```python
from build123d import *

# Parameters (mm, degrees)
BOSS_EXTRUDE1_DEPTH = 25.654
FILLET1_R           = 25.4
FILLET2_R           = 2.54


with BuildPart() as part:
    # Sketch1 → Boss-Extrude1 (new body)
    with BuildSketch(Plane(origin=(0, 0, 0), x_dir=(0, 0, -1), z_dir=(1, 0, 0))):
        Polygon((-8.1595, -12.7), (-6.1595, -12.7), (-6.1595, 0), (6.1595, 0), (6.1595, -25.4), (8.1595, -25.4), (8.1595, 3.175), (-8.1595, 3.175), align=None)
    extrude(amount=BOSS_EXTRUDE1_DEPTH)

    # Fillet1
    # the kernel refuses this fillet: 25.4 mm, written as the material it takes off along each edge
    with BuildSketch(Plane(origin=(-24.69817807, -12.7, 8.1595), x_dir=(0, 0, -1), z_dir=(1, 0, 0))) as fillet1_piece_1:
        with BuildLine():
            CenterArc((25.4, 9.879271228), FILLET1_R, 180, 22.889037196)
            Line((0, 9.879271228), (-0.508, 9.879271228))
            Line((-0.508, 9.879271228), (-0.508, 0))
            Line((-0.508, 0), (0, -0.508))
            ThreePointArc((0, -0.508), (1, -0.508), (1.532, -0.197585425))
            Line((1.532, -0.197585425), (2, 0))
        make_face()
    extrude(amount=75.050356141, mode=Mode.SUBTRACT)
    with BuildSketch(Plane(origin=(-24.69817807, -25.4, -8.1595), x_dir=(0, 0, 1), z_dir=(1, 0, 0))) as fillet1_piece_2:
        with BuildLine():
            CenterArc((25.4, -9.879271228), FILLET1_R, 157.110962804, 22.889037196)
            Line((0, -9.879271228), (-0.508, -9.879271228))
            Line((-0.508, -9.879271228), (-0.508, 0))
            Line((-0.508, 0), (0, 0.508))
            ThreePointArc((0, 0.508), (1, 0.508), (1.532, 0.197585425))
            Line((1.532, 0.197585425), (2, 0))
        make_face()
    extrude(amount=75.050356141, mode=Mode.SUBTRACT)

    # Fillet2
    fillet2_edges = [part.edges().sort_by_distance(p)[0] for p in [
        (12.827, 3.175, 8.1595),
        (12.827, 3.175, -8.1595),
    ]]
    fillet(fillet2_edges, radius=FILLET2_R)


solid = part.part
```
Geometry check sheet. Reference: the model listing, model coordinates, mm. A direction names the side the tool comes from. Round coordinates to 2 decimals unless told otherwise and drop trailing zeros. Order: outer loops, then holes, each group sorted by start corner. A loop starts at its lowest first (then second) coordinate and runs counter-clockwise, first axis right, second up. Notation, with made-up numbers: (77, -7.5) - (82, -7.5) arc R28 ccw to (82, 11.5) - close; hole circle Ø1 at (-32.75, -26.5). An arc over 180 degrees is marked (long way). Use a Markdown table: item, result. Add a question column.
1) Set-up check for faces 5 (the flat face through (13, -6, 6.16)), 6 (the cylindrical face through (13.007, 2.411, 7.435)): record each of +Z, -Z, +X, -X, +Y, -Y from which the full face is reachable in a straight line by a thin tool's end or side.
2) Section check C-C (y = -6.5). Record the cut outline in (x, z).
3) Thickness scan on line 1 along Z through (x, y) = (12.5, -3); line 2 along Z through (x, y) = (23.5, -8); line 3 along Y through (x, z) = (12.75, 5) (3 decimals). Record the ranges inside material, lowest first.
4) Section check D-D (z = 2.75). Record the cut outline in (x, y) (3 decimals).
5) Section check B-B (x = 8). Record the cut outline in (y, z) (1 decimal), then the cut area to 3 significant figures.
6) Mould release check, pull along Z, two halves, no side actions. Record for faces 1 (the flat face through (13, -13, -6.16)), 2 (the flat face through (25.654, 1, -2)), 3 (the cylindrical face through (13.007, 2.451, -7.396)), 4 (the flat face through (13, 0, 0)): released by +Z, released by -Z, zero draft, split by the parting line, or undercut.
7) Section check A-A (y = -0.5). Record the cut outline in (x, z), then the cut area to 3 significant figures.
8) Gauge pin test, flat ends, axial feed: P1, Ø8, axis at y = -20.5, z = -4.5, coming from the +X side; P2, Ø8, axis at x = 22.5, z = -1.5, coming from the -Y side; P3, Ø1, axis at x = 12.5, y = -20, coming from the -Z side; P4, Ø7.5, axis at x = 16, y = -11.5, coming from the +Z side. Record the tip position at first contact, or that the pin passes through.
Established:
| question | item | result |
|---|---|---|
| 1 | face 5 | +X, -X, -Y |
| 1 | face 6 | +Z, +X, -X, +Y |
| 2 | outline | (0, -8.16) - (25.65, -8.16) - (25.65, -6.16) - (0, -6.16) - close; (0, 6.16) - (25.65, 6.16) - (25.65, 7.89) - (0, 7.89) - close |
| 3 | line 1 | -8.16 to -6.16, 6.16 to 8.16 |
| 3 | line 2 | -8.16 to -6.16, 6.16 to 7.63 |
| 3 | line 3 | 0 to 3.175 |
| 4 | outline | (0, 0) - (25.654, 0) - (25.654, 3.175) - (0, 3.175) - close |
| 5 | outline | (-25.4, -6.2) arc R25.4 ccw to (-15.5, -8.2) - (0.6, -8.2) arc R2.5 ccw to (3.2, -5.6) - (3.2, 5.6) arc R2.5 ccw to (0.6, 8.2) - (-2.8, 8.2) arc R25.4 ccw to (-12.7, 6.2) - (0, 6.2) - (0, -6.2) - close |
| 5 | area | 112 mm2 |
| 6 | face 1 | undercut |
| 6 | face 2 | zero draft |
| 6 | face 3 | released by -Z |
| 6 | face 4 | undercut |
| 7 | outline | (0, -8.16) - (25.65, -8.16) - (25.65, -6.16) - (0, -6.16) - close; (0, 6.16) - (25.65, 6.16) - (25.65, 8.16) - (0, 8.16) - close |
| 7 | area | 103 mm2 |
| 8 | P1 | x = 25.65 |
| 8 | P2 | y = 0 |
| 8 | P3 | z = -7.85 |
| 8 | P4 | z = 7.68 |
